from build123d import *

# Parameters (mm, degrees)
SKETCH1_W           = 29.845
SKETCH1_H           = 120
BOSS_EXTRUDE1_DEPTH = 0.4
BOSS_EXTRUDE2_DEPTH = 120
SKETCH2_R           = 1.984375
CUT_EXTRUDE1_DEPTH  = 7.055211633
LPATTERN1_COUNT     = 15
LPATTERN1_PITCH     = 13.75
SKETCH4_R           = 3.5941
CUT_EXTRUDE2_DEPTH  = 2
LPATTERN2_COUNT     = 10
LPATTERN2_PITCH     = 13.75


with BuildPart() as part:
    # Sketch1 → Boss-Extrude1 (new body)
    with BuildSketch(Plane.XY):
        with Locations((14.9225, 60)):
            Rectangle(SKETCH1_W, SKETCH1_H)
    extrude(amount=BOSS_EXTRUDE1_DEPTH)

    # Sketch3 → Boss-Extrude2 (add, through all)
    with BuildSketch(Plane(origin=(0, 120, 0), x_dir=(1, 0, 0), z_dir=(0, 1, 0))):
        with BuildLine():
            Line((29.845, 0), (0, 0))
            ThreePointArc((0, 0), (14.9225, 5.655211633), (29.845, 0))
        make_face()
    extrude(amount=-BOSS_EXTRUDE2_DEPTH)

    # Sketch2 → Cut-Extrude1 (cut, through all)
    with BuildSketch(Plane.XY.offset(0.4)):
        with Locations((14.9225, 0)):
            Circle(SKETCH2_R)
    cut_extrude1 = extrude(amount=-CUT_EXTRUDE1_DEPTH, mode=Mode.SUBTRACT)

    # LPattern1: Cut-Extrude1 ×15
    with Locations(*[(0, i * LPATTERN1_PITCH, 0) for i in range(1, LPATTERN1_COUNT)]):
        add(cut_extrude1, mode=Mode.SUBTRACT)

    # Sketch4 → Cut-Extrude2 (cut)
    with BuildSketch(Plane.XY.offset(0.4)):
        with Locations((14.9225, 0)):
            Circle(SKETCH4_R)
    cut_extrude2 = extrude(amount=-CUT_EXTRUDE2_DEPTH, mode=Mode.SUBTRACT)

    # LPattern2: Cut-Extrude2 ×10
    with Locations(*[(0, i * LPATTERN2_PITCH, 0) for i in range(1, LPATTERN2_COUNT)]):
        add(cut_extrude2, mode=Mode.SUBTRACT)


solid = part.part
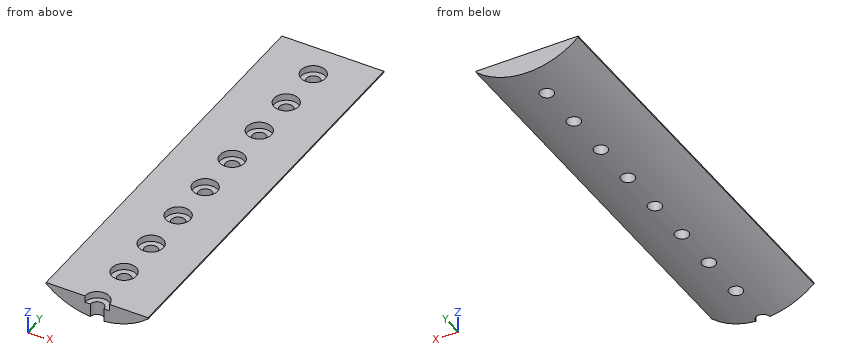
Check sheet for the modelled part. Datum: model origin and axes. Units: mm. Round coordinates to 2 decimals unless told otherwise and drop trailing zeros. Write each loop counter-clockwise with the first axis right and the second up, starting at its lowest first coordinate (ties: lowest second). Pieces come first, ordered by that corner, then holes. Notation, with made-up numbers: (79, 34.25) - (100, 34.25) arc R27 cw to (100, 56.25) - close; hole circle Ø5 at (-22.75, -37). An arc over 180 degrees is marked (long way). Return JSON: item names as keys, results as strings.
Q1. Depth check by flat-ended pin: P1, Ø4.5, axis at x = 14.92, y = 68.75, coming from the +Z side; P2, Ø11.5, axis at x = 14.92, y = 82.5, coming from the -Z side; P3, Ø4, axis at x = 18.5, y = 14.5, coming from the -Z side; P4, Ø3, axis at y = 82.5, z = -2.5, coming from the -X side. Enter the tip coordinate at first touch or a pass-through.
Returned:
{"P1": "stops at z = -1.6", "P2": "stops at z = -5.66", "P3": "stops at z = -5.6", "P4": "stops at x = 1.21"}
Q2. Cross-section at A-A (y = 13.75). Record the boundary of the cut face in (x, z) (1 decimal).
Returned:
{"outline": "(0, 0) arc R22.5 ccw to (12.9, -5.6) - (12.9, -1.6) - (11.3, -1.6) - (11.3, 0.4) - (0, 0.4) - close; (16.9, -5.6) arc R22.5 ccw to (29.8, 0) - (29.8, 0.4) - (18.5, 0.4) - (18.5, -1.6) - (16.9, -1.6) - close"}
Q3. Cross-section at C-C (y = 64). Record the boundary of the cut face in (x, z) (1 decimal).
Returned:
{"outline": "(0, 0) arc R22.5 ccw to (29.8, 0) - (29.8, 0.4) - (0, 0.4) - close"}
Q4. Scan lines: L1, parallel to X at y = 27.5, z = -3.2; L2, parallel to X at y = 96.25, z = -3.8; L3, parallel to Z at x = 13.25, y = 84. Record each from-to range of solid material in increasing order. Write a range as from..to.
Returned:
{"L1": "x = 4.7..12.94, 16.91..25.15", "L2": "x = 5.97..12.94, 16.91..23.87", "L3": "z = -5.59..-1.6"}
Q5. Cross-section at B-B (z = -3.75). Give the number of separate pieces and of enclosed holes in the cut face, then the cut area to 3 significant figures.
Returned:
{"separate pieces": "1", "enclosed holes": "8", "area": "2,070 mm²"}
